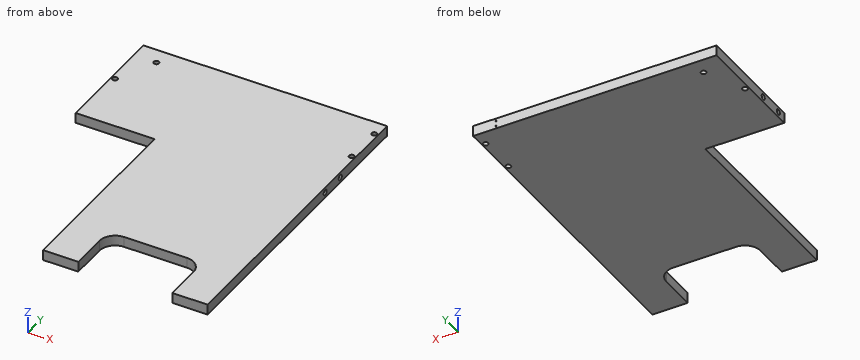
from build123d import *

# Parameters (mm, degrees)
EXTRUDE_1_DEPTH     = 20
SKETCH_2_R          = 5
CUT_EXTRUDE_1_DEPTH = 757.029761319
SKETCH_3_R          = 5.15
CUT_EXTRUDE_2_DEPTH = 20
CUT_EXTRUDE_START   = -20
SKETCH_4_R          = 5.15
CUT_EXTRUDE_3_DEPTH = 20
SKETCH_5_R          = 1.25
CUT_EXTRUDE_4_DEPTH = 10


with BuildPart() as part:
    # 草图1 → 凸台-拉伸1 (new body)
    with BuildSketch(Plane.XY):
        Polygon((0, 0), (466, 0), (466, -595), (151, -595), (151, -225), (0, -225), align=None)
    extrude(amount=-EXTRUDE_1_DEPTH)

    # 草图2 → 切除-拉伸1 (cut, through all)
    with BuildSketch(Plane.XY):
        with Locations((43.2, -32)):
            Circle(SKETCH_2_R)
        with Locations((459, -30)):
            Circle(SKETCH_2_R)
        with Locations((459, -105)):
            Circle(SKETCH_2_R)
        with Locations((7.2, -107)):
            Circle(SKETCH_2_R)
        with BuildLine():
            Line((218.5, -595), (218.5, -525))
            ThreePointArc((218.5, -525), (227.286796564, -503.786796564), (248.5, -495))
            Line((248.5, -495), (368.5, -495))
            ThreePointArc((368.5, -495), (389.713203436, -503.786796564), (398.5, -525))
            Line((398.5, -525), (398.5, -595))
            Line((398.5, -595), (218.5, -595))
        make_face()
    extrude(amount=-CUT_EXTRUDE_1_DEPTH, mode=Mode.SUBTRACT)

    # 草图3 → 切除-拉伸2 (cut)
    with BuildSketch(Plane.ZY):
        with Locations((-10, -155)):
            Circle(SKETCH_3_R)
        with Locations((-10, -205)):
            Circle(SKETCH_3_R)
    extrude(amount=-CUT_EXTRUDE_2_DEPTH, mode=Mode.SUBTRACT)

    # 草图4 → 切除-拉伸3 (cut)
    with BuildSketch(Plane(origin=(466, 0, 0), x_dir=(0, 0, -1), z_dir=(1, 0, 0)).offset(CUT_EXTRUDE_START)):
        with Locations(Location((10, -155, 0), (0, 0, 180))):
            Circle(SKETCH_4_R)
        with Locations(Location((10, -205, 0), (0, 0, 180))):
            Circle(SKETCH_4_R)
    extrude(amount=CUT_EXTRUDE_3_DEPTH, mode=Mode.SUBTRACT)

    # 草图5 → 切除-拉伸4 (cut)
    with BuildSketch(Plane(origin=(0, 0, 0), x_dir=(1, 0, 0), z_dir=(0, 1, 0))):
        with Locations(Location((422, 15, 0), (0, 0, 270))):
            Circle(SKETCH_5_R)
        with Locations(Location((422, 5, 0), (0, 0, 270))):
            Circle(SKETCH_5_R)
    extrude(amount=-CUT_EXTRUDE_4_DEPTH, mode=Mode.SUBTRACT)


solid = part.part
Input: part model. Units: mm. Frame: model coordinates. Round coordinates to 2 decimals unless told otherwise and drop trailing zeros. Order: outer loops, then holes, each group sorted by start corner. A loop starts at its lowest first (then second) coordinate and runs counter-clockwise, first axis right, second up.
1. Pin query (flat end, axial travel): P1, Ø1, axis at y = -496, z = -13.5, coming from the -X side; P2, Ø3, axis at y = -206, z = -8.5, coming from the +X side; P3, Ø10, axis at x = 61.5, z = -13, coming from the -Y side; P4, Ø8, axis at x = 43.2, y = -32, coming from the -Z side. Return the tip coordinate at first contact, or that it passes through.
The answers:
P1: stops at x = 151
P2: stops at x = 446
P3: stops at y = -225
P4: passes through
2. Cut plane C-C, the plane x = 276.5. Output: boundary loops of the cut face in (y, z), then the cut area to 3 significant figures.
The answers:
outline: (-495, -20) - (0, -20) - (0, 0) - (-495, 0) - close
area: 9,900 mm2
3. Cut plane A-A, the plane z = -10. State how many separate pieces and enclosed holes the cut face has, then the cut area to 3 significant figures.
The answers:
separate pieces: 1
enclosed holes: 4
area: 203,000 mm2
4. Material intervals for line 1 (Z direction, x = 422, y = -3.25); line 2 (Y direction, x = 451.75, z = -10); line 3 (Y direction, x = 459, z = -10), sorted ascending.
The answers:
line 1: z = -20 to -16.25, -13.75 to -6.25, -3.75 to 0
line 2: y = -595 to -210.15, -199.85 to -160.15, -149.85 to 0
line 3: y = -595 to -210.15, -199.85 to -160.15, -149.85 to -110, -100 to -35, -25 to 0
5. Cut plane B-B, the plane y = -268.5. Output: boundary loops of the cut face in (x, z), then the cut area to 3 significant figures.
The answers:
outline: (151, -20) - (466, -20) - (466, 0) - (151, 0) - close
area: 6,300 mm2
